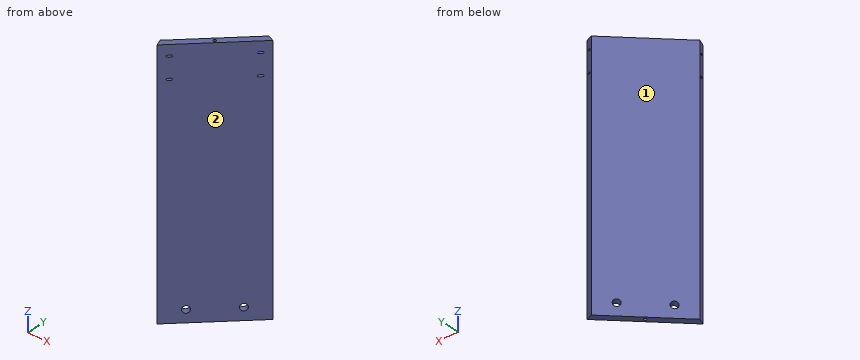
```python
from build123d import *

# Parameters (mm, degrees)
F1_DEPTH       = 240
F2_DEPTH       = 240
F3_DEPTH       = 240
F4_DEPTH       = 240
F9_D           = 6.6
F9_DEPTH       = 12
F9_TIP         = 1.9828400428
F9_ON_F5_D     = 6.6
F9_ON_F5_DEPTH = 12
F9_ON_F5_TIP   = 1.9828400428
F9_ON_F6_D     = 6.6
F9_ON_F6_DEPTH = 12
F9_ON_F6_TIP   = 1.9828400428
F9_ON_F7_D     = 6.6
F9_ON_F7_DEPTH = 12
F9_ON_F7_TIP   = 1.9828400428
F13_D          = 2.7051
F13_ON_F10_D   = 2.7051
F13_ON_F12_D   = 2.7051
F17_D          = 1.9939
F17_ON_F14_D   = 1.9939


with BuildPart() as f1:
    # F0 (on Top) → F1 (new body)
    with BuildSketch(Plane.XY):
        Polygon((-180, 60), (-120, 0), (-117.3697438789, 6.35), (-173.65, 62.6302561211), align=None)
    extrude(amount=F1_DEPTH)

    # F9 on F5
    with Locations(Plane(origin=(-60, -60, 0), x_dir=(0.7071067812, -0.7071067812, 0), z_dir=(-0.7071067812, -0.7071067812, 0))):
        with Locations((-106.066017178, 11.51), (-148.4924240492, 11.51)):
            Hole(F9_ON_F5_D / 2, depth=F9_ON_F5_DEPTH)
            with Locations((0, 0, -(F9_ON_F5_DEPTH + F9_ON_F5_TIP / 2))):  # 118° drill point
                Cone(0, F9_ON_F5_D / 2, F9_ON_F5_TIP, mode=Mode.SUBTRACT)

    # F13 on F10 (through all)
    with Locations(Plane(origin=(0, 0, 0), x_dir=(1, 0, 0), z_dir=(0, 0, -1))):
        with Locations((-147.7549359697, -32.2450640303)):
            Hole(F13_ON_F10_D / 2)


with BuildPart() as f2:
    # F0 (on Top) → F2 (new body)
    with BuildSketch(Plane.XY):
        Polygon((-120, 280), (-180, 220), (-173.65, 217.3697438789), (-117.3697438789, 273.65), align=None)
    extrude(amount=F2_DEPTH)

    # F9
    with Locations(Plane(origin=(-200, 200, 0), x_dir=(-0.7071067812, -0.7071067812, 0), z_dir=(-0.7071067812, 0.7071067812, 0))):
        with Locations((-91.9238815543, 11.51), (-49.4974746831, 11.51)):
            Hole(F9_D / 2, depth=F9_DEPTH)
            with Locations((0, 0, -(F9_DEPTH + F9_TIP / 2))):  # 118° drill point
                Cone(0, F9_D / 2, F9_TIP, mode=Mode.SUBTRACT)

    # F13 on F12 (through all)
    with Locations(Plane(origin=(0, 0, 0), x_dir=(1, 0, 0), z_dir=(0, 0, -1))):
        with Locations((-147.7549359697, -247.7549359697)):
            Hole(F13_ON_F12_D / 2)


with BuildPart() as f3:
    # F0 (on Top) → F3 (new body)
    with BuildSketch(Plane.XY):
        Polygon((173.65, 217.3697438789), (180, 220), (120, 280), (117.3697438789, 273.65), align=None)
    extrude(amount=F3_DEPTH)

    # F9 on F7
    with Locations(Plane(origin=(200, 200, 0), x_dir=(-0.7071067812, 0.7071067812, 0), z_dir=(0.7071067812, 0.7071067812, 0))):
        with Locations((49.4974746831, 11.51), (91.9238815543, 11.51)):
            Hole(F9_ON_F7_D / 2, depth=F9_ON_F7_DEPTH)
            with Locations((0, 0, -(F9_ON_F7_DEPTH + F9_ON_F7_TIP / 2))):  # 118° drill point
                Cone(0, F9_ON_F7_D / 2, F9_ON_F7_TIP, mode=Mode.SUBTRACT)


with BuildPart() as f4:
    # F0 (on Top) → F4 (new body)
    with BuildSketch(Plane.XY):
        Polygon((117.3697438789, 6.35), (120, 0), (180, 60), (173.65, 62.6302561211), align=None)
    extrude(amount=F4_DEPTH)

    # F9 on F6
    with Locations(Plane(origin=(60, -60, 0), x_dir=(0.7071067812, 0.7071067812, 0), z_dir=(0.7071067812, -0.7071067812, 0))):
        with Locations((148.4924240492, 11.51), (106.066017178, 11.51)):
            Hole(F9_ON_F6_D / 2, depth=F9_ON_F6_DEPTH)
            with Locations((0, 0, -(F9_ON_F6_DEPTH + F9_ON_F6_TIP / 2))):  # 118° drill point
                Cone(0, F9_ON_F6_D / 2, F9_ON_F6_TIP, mode=Mode.SUBTRACT)

    # F13 (through all)
    with Locations(Plane(origin=(0, 0, 0), x_dir=(1, 0, 0), z_dir=(0, 0, -1))):
        with Locations((147.7549359697, -32.2450640303)):
            Hole(F13_D / 2)

    # F17 (through all)
    with Locations(Plane(origin=(47.5735931288, 114.8528137424, 0), x_dir=(-0.9238795325, 0.3826834324, 0), z_dir=(0.3826834324, 0.9238795325, 0))):
        with Locations((-139.9007146742, 230), (-139.9007146742, 210)):
            Hole(F17_D / 2)

    # F17 on F14 (through all)
    with Locations(Plane(origin=(102.4264068712, 42.4264068712, 0), x_dir=(0.3826834324, -0.9238795325, 0), z_dir=(-0.9238795325, -0.3826834324, 0))):
        with Locations((42.4854166479, 230), (42.4854166479, 210)):
            Hole(F17_ON_F14_D / 2)


solid = f4.part
```
Part model, mm, in its own coordinate system. Face numbers are marked on the shaded views. Give positions to 0.01 mm unless a question says otherwise; leave off trailing zeros. Order: outer loops, then holes, each group sorted by start corner. A loop starts at its lowest first (then second) coordinate and runs counter-clockwise, first axis right, second up. Notation, with made-up numbers: M 44.25,26 L 93.25,26 A28 ccw 93.25,51 Z; hole C 71,49 d2. An arc over 180 degrees is marked long. Use a Markdown table: item, result. Add a question column.
(1) Drop flat-ended pins along their axis: P1, Ø10, axis at x = 165.5, z = 33.5, coming from the -Y side; P2, Ø4, axis at y = 55.5, z = 58.5, coming from the +X side; P3, Ø2, axis at x = 142, z = 215.5, coming from the +Y side; P4, Ø3, axis at x = 148.5, y = 40.5, coming from the -Z side. Give the stop position or say it passes through.
(2) Mould opens along X. For the marked faces 1 and 2 say: +X half, -X half, draft (parallel to the pull), parting line (faces both ways), or undercut.
(3) Saw through at A-A, the plane z = 129.5. Give the cut face in (x, y), and give its area (3 significant figures).
(4) Probe line 1 along Z through (x, y) = (122.5, 4.5); line 2 along Y through (x, z) = (154, 24); line 3 along X through (y, z) = (55.5, 125.5). List the from-to ranges inside material, lowest first. Write a range as [from, to].
(5) Saw through at B-B, the plane y = 39. Give the cut face in (x, z).
(6) Saw through at C-C, the plane x = 155. Give the cut face in (y, z), and give its area (3 significant figures).
Answer key:
| question | item | result |
|---|---|---|
| 1 | P1 | y = 40.5 |
| 1 | P2 | x = 177.5 |
| 1 | P3 | y = 31.98 |
| 1 | P4 | through |
| 2 | face 1 | -X half |
| 2 | face 2 | +X half |
| 3 | outline | M 117.37,6.35 L 120,0 L 180,60 L 173.65,62.63 Z; hole C 147.75,32.25 d2.71 |
| 3 | area | 516 mm^2 |
| 4 | line 1 | [0, 209.03], [210.97, 229.03], [230.97, 240] |
| 4 | line 2 | [34, 42.98] |
| 4 | line 3 | [166.52, 175.5] |
| 5 | outline | M 150.02,0 L 159,0 L 159,240 L 150.02,240 Z |
| 6 | outline | M 35,0 L 43.98,0 L 43.98,240 L 35,240 Z |
| 6 | area | 2,160 mm^2 |
